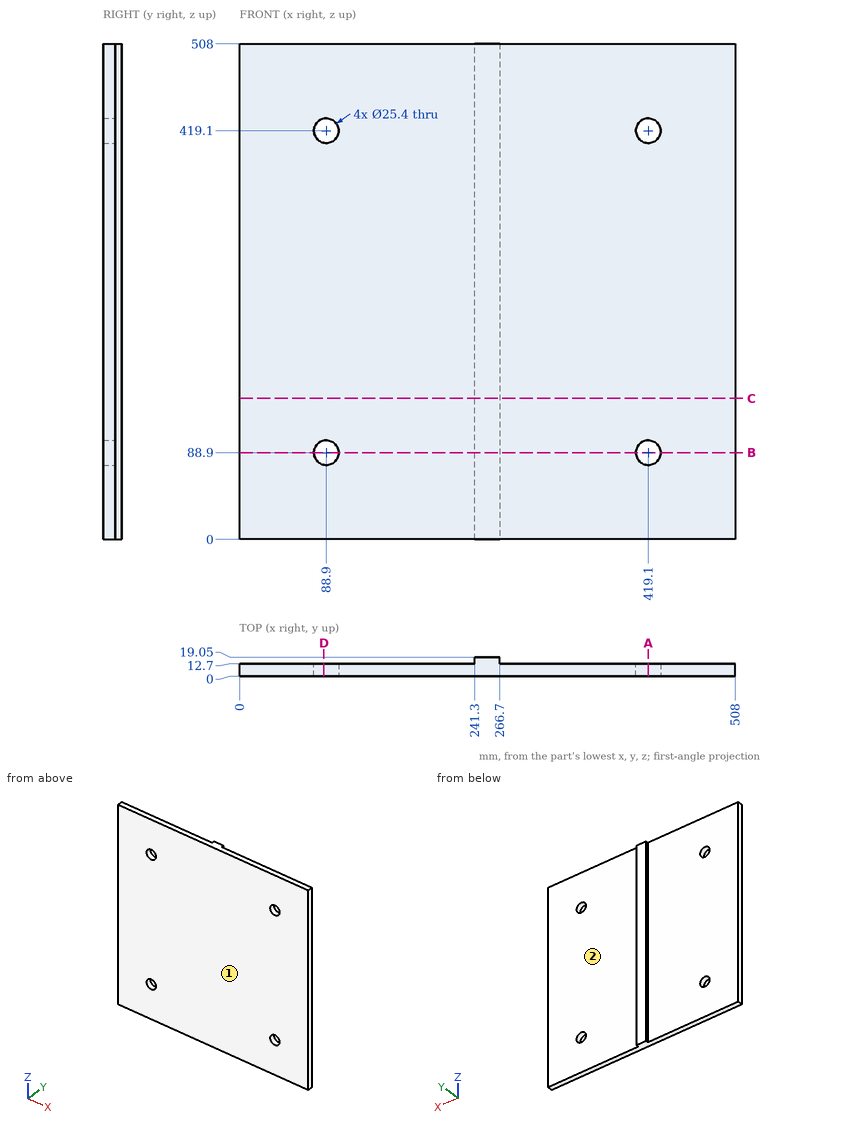
The figure shows three views and two pictorial views of one solid part (mm, origin at its lowest corner). Answer the questions. Give positions to 0.01 mm unless a question says otherwise; leave off trailing zeros. Write each loop counter-clockwise with the first axis right and the second up, starting at its lowest first coordinate (ties: lowest second). Pieces come first, ordered by that corner, then holes. Notation, with made-up numbers: (-12.75, 82.5) - (-2.75, 82.5) arc R33 cw to (-2.75, 112.5) - close; hole circle Ø3 at (42, 73). An arc over 180 degrees is marked (long way). Use one line per item in the form item = value. Start each with the question number.
1) The mould has two halves that part along Y. Classify the marked faces 1 and 2: pulls with the +Y half, pulls with the -Y half, needs draft (parallel to the pull), parting line crosses it, or undercut.
2) Find section D-D on x = 86.5. Determine the outline of the cut face in (y, z), plus the area to 3 significant figures.
3) Find section A-A on x = 419.1. Determine the outline of the cut face in (y, z), plus the area to 3 significant figures.
4) Find section B-B on z = 88.9. Determine the outline of the cut face in (x, y), plus the area to 3 significant figures.
5) Find section C-C on z = 144.5. Determine the outline of the cut face in (x, y), plus the area to 3 significant figures.
6) Consider line 1 along Z through (x, y) = (419.1, 3.25); line 2 along Y through (x, z) = (383, 304.5). Determine where each line is inside the solid, lowest interval first. Write a range as from..to.
7) Flat-ended cylindrical pins translate along their axes: pin 1 Ø2 at (x, y) = (440, 6) entering from -Z; pin 2 Ø5 at (x, z) = (78.5, 85.5) entering from +Y; pin 3 Ø3 at (y, z) = (17, 342) entering from -X; pin 4 Ø7 at (y, z) = (16.5, 301.5) entering from +X. Find the tip coordinate at first contact, or state that the pin passes through.
Geometry results:
q1.face_1 = pulls with the -Y half
q1.face_2 = pulls with the +Y half
q2.outline = (0, 0) - (12.7, 0) - (12.7, 76.43) - (0, 76.43) - close; (0, 101.37) - (12.7, 101.37) - (12.7, 406.63) - (0, 406.63) - close; (0, 431.57) - (12.7, 431.57) - (12.7, 508) - (0, 508) - close
q2.area = 5,820 mm2
q3.outline = (0, 0) - (12.7, 0) - (12.7, 76.2) - (0, 76.2) - close; (0, 101.6) - (12.7, 101.6) - (12.7, 406.4) - (0, 406.4) - close; (0, 431.8) - (12.7, 431.8) - (12.7, 508) - (0, 508) - close
q3.area = 5,810 mm2
q4.outline = (0, 0) - (76.2, 0) - (76.2, 12.7) - (0, 12.7) - close; (101.6, 0) - (406.4, 0) - (406.4, 12.7) - (266.7, 12.7) - (266.7, 19.05) - (241.3, 19.05) - (241.3, 12.7) - (101.6, 12.7) - close; (431.8, 0) - (508, 0) - (508, 12.7) - (431.8, 12.7) - close
q4.area = 5,970 mm2
q5.outline = (0, 0) - (508, 0) - (508, 12.7) - (266.7, 12.7) - (266.7, 19.05) - (241.3, 19.05) - (241.3, 12.7) - (0, 12.7) - close
q5.area = 6,610 mm2
q6.line_1 = 0..76.2, 101.6..406.4, 431.8..508
q6.line_2 = 0..12.7
q7.pin_1 = 0
q7.pin_2 = 12.7
q7.pin_3 = 241.3
q7.pin_4 = 266.7
